The drawing under review shows one solid part. Ordinate dimensions are in mm from its lowest x, y, z. Coordinates: 2 decimals unless noted, no trailing zeros. Order: outer loops, then holes, each group sorted by start corner. A loop starts at its lowest first (then second) coordinate and runs counter-clockwise, first axis right, second up. Notation, with made-up numbers: (6, -3.75) -> (40, -3.75) arc R7 cw to (40, 1.25) -> close; hole circle Ø1 at (57.5, 25.25). An arc over 180 degrees is marked (long way). Write item = value, one per line.
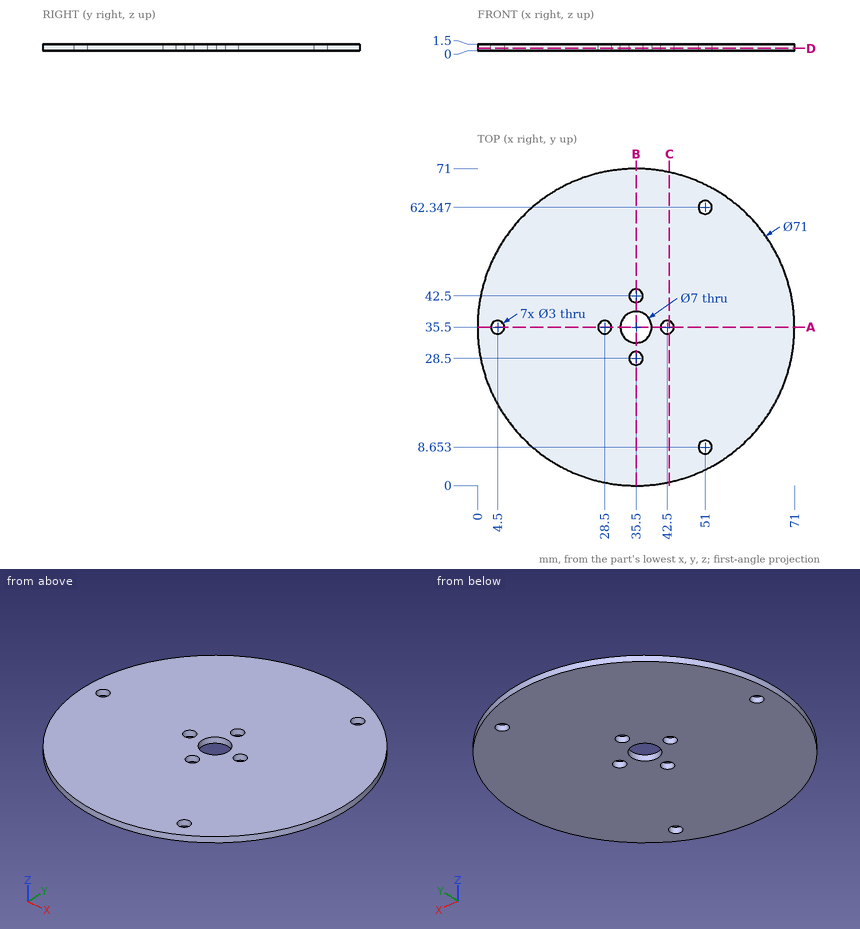
(1) For L1, parallel to Y at x = 35.5, z = 0.95; L2, parallel to Y at x = 51, z = 1.05; L3, parallel to X at y = 9, z = 0.7, list the stretches that pass through material, from the lowest coordinate up.
Report:
L1 = 0 to 27, 30 to 32, 39 to 41, 44 to 71
L2 = 3.56 to 7.15, 10.15 to 60.85, 63.85 to 67.44
L3 = 11.88 to 49.54, 52.46 to 59.12
(2) We need section B-B (x = 35.5). Write out the cut boundary in (y, z).
Report:
outline = (0, 0) -> (27, 0) -> (27, 1.5) -> (0, 1.5) -> close; (30, 0) -> (32, 0) -> (32, 1.5) -> (30, 1.5) -> close; (39, 0) -> (41, 0) -> (41, 1.5) -> (39, 1.5) -> close; (44, 0) -> (71, 0) -> (71, 1.5) -> (44, 1.5) -> close
(3) We need section C-C (x = 43). Write out the cut boundary in (y, z).
Report:
outline = (0.8, 0) -> (34.09, 0) -> (34.09, 1.5) -> (0.8, 1.5) -> close; (36.91, 0) -> (70.2, 0) -> (70.2, 1.5) -> (36.91, 1.5) -> close
(4) We need section A-A (y = 35.5). Write out the cut boundary in (x, z).
Report:
outline = (0, 0) -> (3, 0) -> (3, 1.5) -> (0, 1.5) -> close; (6, 0) -> (27, 0) -> (27, 1.5) -> (6, 1.5) -> close; (30, 0) -> (32, 0) -> (32, 1.5) -> (30, 1.5) -> close; (39, 0) -> (41, 0) -> (41, 1.5) -> (39, 1.5) -> close; (44, 0) -> (71, 0) -> (71, 1.5) -> (44, 1.5) -> close
(5) We need section D-D (z = 0.5). Give the number of separate pieces and of enclosed holes in the cut face, and give its area (3 significant figures).
Report:
separate_pieces = 1
enclosed_holes = 8
area = 3,870 mm²
